Source: CAD feature listing. Evaluate the final solid. Frame: model axes, mm. Face numbers are marked on the shaded views. A direction names the side the tool comes from. Coordinates: 2 decimals unless noted, no trailing zeros. Order: outer loops, then holes, each group sorted by start corner. A loop starts at its lowest first (then second) coordinate and runs counter-clockwise, first axis right, second up.
Item 1: Ray query, line 1 (X direction, y = 6.5, z = 19.75); line 2 (X direction, y = 14.5, z = 8); line 3 (X direction, y = -17, z = 13.5). Return the intervals inside material, ascending.
Item 2: Section D-D on x = -48. Return the cut outline in (y, z), then the cut area to 3 significant figures.
Item 3: Section A-A on z = 5.25. Return the cut outline in (x, y), then the cut area to 3 significant figures.
Item 4: Contact query for flat-ended pins moving along their axis: P1, Ø12.5, axis at x = 45.5, z = 15.5, coming from the +Y side; P2, Ø2, axis at x = -30.5, z = 6.5, coming from the +Y side; P3, Ø12, axis at x = -31.5, z = 16.5, coming from the +Y side. Output: stop coordinate, or through.
Item 5: Section B-B on x = 41.5. Return the cut outline in (y, z).
Item 6: Section C-C on y = -4. Return the cut outline in (x, z), then the cut area to 3 significant figures.
Item 7: Reachability of the marked faces 1 and 2 from +Z, -Z, +X, -X, +Y, -Y: full face, straight path, thin tool, end or side. Return the list, or none.
Item 8: Mould query, pull axis Y, two halves, no side actions, for the marked faces 3, 4 and 5. Classes: released by +Y, released by -Y, zero draft, split by the parting line, or undercut.
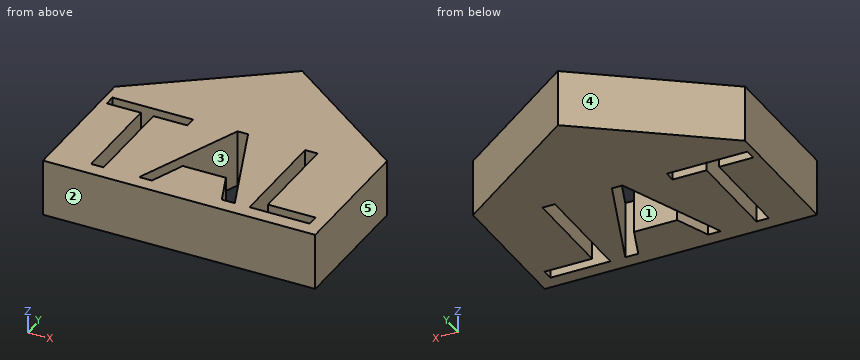
from build123d import *

# Parameters (mm, degrees)
F1_DEPTH = 25
F0_W     = 119.9337523431
F0_H     = 61.4086027442
F2_DEPTH = 25
F3_DEPTH = 25


with BuildPart() as f1:
    # F0 (on Top) → F1 (new body)
    with BuildSketch(Plane.XY):
        Polygon((-59.9668761715, 30.7043013721), (59.9668761715, 30.7043013721), (0, 74.5766162872), align=None)
    extrude(amount=F1_DEPTH)

    # F0 (on Top) → F2 (join)
    with BuildSketch(Plane.XY):
        Rectangle(F0_W, F0_H)
        Polygon((-36.5568330017, 18.276524249), (-36.5568330017, -24.3145190179), (-42.0769316042, -24.3145190179), (-42.0769316042, 18.276524249), (-57.1194601879, 18.276524249), (-57.1194601879, 23.1832785624), (-21.514304418, 23.1832785624), (-21.514304418, 18.276524249), align=None, mode=Mode.SUBTRACT)
        Polygon((21.2118825059, -24.3145190179), (15.4942662508, -24.3145190179), (9.5791323434, -9.2096164388), (-9.4553319529, -9.2096164388), (-15.2976961989, -24.3145190179), (-20.8905644629, -24.3145190179), (-2.1159918146, 23.3807962149), (2.5308708508, 23.3807962149), align=None, mode=Mode.SUBTRACT)
        Polygon((54.2181217962, -24.3145190179), (27.7403607025, -24.3145190179), (27.7403607025, 23.1832785624), (33.2604593051, 23.1832785624), (33.2604593051, -19.3142037113), (54.2181217962, -19.3142037113), align=None, mode=Mode.SUBTRACT)
        Polygon((-59.9668761715, 30.7043013721), (59.9668761715, 30.7043013721), (0, 74.5766162872), align=None)
    extrude(amount=F2_DEPTH)

    # F0 (on Top) → F3 (join)
    with BuildSketch(Plane.XY):
        Rectangle(F0_W, F0_H)
        Polygon((-36.5568330017, 18.276524249), (-36.5568330017, -24.3145190179), (-42.0769316042, -24.3145190179), (-42.0769316042, 18.276524249), (-57.1194601879, 18.276524249), (-57.1194601879, 23.1832785624), (-21.514304418, 23.1832785624), (-21.514304418, 18.276524249), align=None, mode=Mode.SUBTRACT)
        Polygon((21.2118825059, -24.3145190179), (15.4942662508, -24.3145190179), (9.5791323434, -9.2096164388), (-9.4553319529, -9.2096164388), (-15.2976961989, -24.3145190179), (-20.8905644629, -24.3145190179), (-2.1159918146, 23.3807962149), (2.5308708508, 23.3807962149), align=None, mode=Mode.SUBTRACT)
        Polygon((54.2181217962, -24.3145190179), (27.7403607025, -24.3145190179), (27.7403607025, 23.1832785624), (33.2604593051, 23.1832785624), (33.2604593051, -19.3142037113), (54.2181217962, -19.3142037113), align=None, mode=Mode.SUBTRACT)
    extrude(amount=F3_DEPTH)


solid = f1.part
Answer list:
1. line 1: x = -59.97 to -42.08, -36.56 to -8.76, 9.14 to 27.74, 33.26 to 59.97
1. line 2: x = -59.97 to -42.08, -36.56 to -5.61, 6.01 to 27.74, 33.26 to 59.97
1. line 3: x = -59.97 to -42.08, -36.56 to -18.01, -12.47 to 12.63, 18.35 to 27.74, 33.26 to 59.97
2. outline: (-30.7, 0) - (18.28, 0) - (18.28, 25) - (-30.7, 25) - close; (23.18, 0) - (39.46, 0) - (39.46, 25) - (23.18, 25) - close
2. area: 1,630 mm2
3. outline: (-59.97, -30.7) - (59.97, -30.7) - (59.97, 30.7) - (0, 74.58) - (-59.97, 30.7) - close; hole (-57.12, 18.28) - (-42.08, 18.28) - (-42.08, -24.31) - (-36.56, -24.31) - (-36.56, 18.28) - (-21.51, 18.28) - (-21.51, 23.18) - (-57.12, 23.18) - close; hole (-20.89, -24.31) - (-15.3, -24.31) - (-9.46, -9.21) - (9.58, -9.21) - (15.49, -24.31) - (21.21, -24.31) - (2.53, 23.38) - (-2.12, 23.38) - close; hole (27.74, -24.31) - (54.22, -24.31) - (54.22, -19.31) - (33.26, -19.31) - (33.26, 23.18) - (27.74, 23.18) - close
3. area: 8,480 mm2
4. P1: stops at y = 45.86
4. P2: stops at y = 52.99
4. P3: stops at y = 55.92
5. outline: (-30.7, 0) - (-24.31, 0) - (-24.31, 25) - (-30.7, 25) - close; (-19.31, 0) - (44.21, 0) - (44.21, 25) - (-19.31, 25) - close
6. outline: (-59.97, 0) - (-42.08, 0) - (-42.08, 25) - (-59.97, 25) - close; (-36.56, 0) - (-12.89, 0) - (-12.89, 25) - (-36.56, 25) - close; (13.26, 0) - (27.74, 0) - (27.74, 25) - (13.26, 25) - close; (33.26, 0) - (59.97, 0) - (59.97, 25) - (33.26, 25) - close
6. area: 2,070 mm2
7. face 1: +Z, -Z
7. face 2: +Z, -Z, +X, -X, -Y
8. face 3: undercut
8. face 4: released by +Y
8. face 5: zero draft
